from build123d import *

# Parameters (mm, degrees)
F1_DEPTH = 3.302
F2_DEPTH = 2.54
F3_R     = 5.715
F3_R_2   = 2.8702
F3_R_3   = 2.1123361497
F4_DEPTH = 3.303
F5_R     = 1.26999


# Not quite as in the source:
# - a fillet or chamfer is up to 0.001 mm smaller than in the source, because OpenCascade refuses the exact size


with BuildPart() as f1:
    # F0 (on Top) → F1 (new body)
    with BuildSketch(Plane.XY):
        with BuildLine():
            Line((86.5189202702, -3.8629329861), (10.3189202702, -3.8629329861))
            ThreePointArc((10.3189202702, -3.8629329861), (8.0738562399, -4.7928689558), (7.1439202702, -7.0379329861))
            Line((7.1439202702, -7.0379329861), (7.1439202702, -32.4379329861))
            ThreePointArc((7.1439202702, -32.4379329861), (8.0738562399, -34.6829970164), (10.3189202702, -35.6129329861))
            Line((10.3189202702, -35.6129329861), (86.5189202702, -35.6129329861))
            ThreePointArc((86.5189202702, -35.6129329861), (88.7639843005, -34.6829970164), (89.6939202702, -32.4379329861))
            Line((89.6939202702, -32.4379329861), (89.6939202702, -7.0379329861))
            ThreePointArc((89.6939202702, -7.0379329861), (88.7639843005, -4.7928689558), (86.5189202702, -3.8629329861))
        make_face()
        with BuildLine():
            Line((83.9789202702, -33.0729329861), (12.8589202702, -33.0729329861))
            ThreePointArc((12.8589202702, -33.0729329861), (10.6138562399, -32.1429970164), (9.6839202702, -29.8979329861))
            Line((9.6839202702, -29.8979329861), (9.6839202702, -9.5779329861))
            ThreePointArc((9.6839202702, -9.5779329861), (10.6138562399, -7.3328689558), (12.8589202702, -6.4029329861))
            Line((12.8589202702, -6.4029329861), (83.9789202702, -6.4029329861))
            ThreePointArc((83.9789202702, -6.4029329861), (86.2239843005, -7.3328689558), (87.1539202702, -9.5779329861))
            Line((87.1539202702, -9.5779329861), (87.1539202702, -29.8979329861))
            ThreePointArc((87.1539202702, -29.8979329861), (86.2239843005, -32.1429970164), (83.9789202702, -33.0729329861))
        make_face(mode=Mode.SUBTRACT)
        with BuildLine():
            ThreePointArc((9.6839202702, -29.8979329861), (10.6138562399, -32.1429970164), (12.8589202702, -33.0729329861))
            Line((12.8589202702, -33.0729329861), (83.9789202702, -33.0729329861))
            ThreePointArc((83.9789202702, -33.0729329861), (86.2239843005, -32.1429970164), (87.1539202702, -29.8979329861))
            Line((87.1539202702, -29.8979329861), (87.1539202702, -9.5779329861))
            ThreePointArc((87.1539202702, -9.5779329861), (86.2239843005, -7.3328689558), (83.9789202702, -6.4029329861))
            Line((83.9789202702, -6.4029329861), (12.8589202702, -6.4029329861))
            ThreePointArc((12.8589202702, -6.4029329861), (10.6138562399, -7.3328689558), (9.6839202702, -9.5779329861))
            Line((9.6839202702, -9.5779329861), (9.6839202702, -29.8979329861))
        make_face()
    extrude(amount=-F1_DEPTH)

    # F0 (on Top) → F2 (join)
    with BuildSketch(Plane.XY):
        with BuildLine():
            Line((86.5189202702, -3.8629329861), (10.3189202702, -3.8629329861))
            ThreePointArc((10.3189202702, -3.8629329861), (8.0738562399, -4.7928689558), (7.1439202702, -7.0379329861))
            Line((7.1439202702, -7.0379329861), (7.1439202702, -32.4379329861))
            ThreePointArc((7.1439202702, -32.4379329861), (8.0738562399, -34.6829970164), (10.3189202702, -35.6129329861))
            Line((10.3189202702, -35.6129329861), (86.5189202702, -35.6129329861))
            ThreePointArc((86.5189202702, -35.6129329861), (88.7639843005, -34.6829970164), (89.6939202702, -32.4379329861))
            Line((89.6939202702, -32.4379329861), (89.6939202702, -7.0379329861))
            ThreePointArc((89.6939202702, -7.0379329861), (88.7639843005, -4.7928689558), (86.5189202702, -3.8629329861))
        make_face()
        with BuildLine():
            Line((83.9789202702, -33.0729329861), (12.8589202702, -33.0729329861))
            ThreePointArc((12.8589202702, -33.0729329861), (10.6138562399, -32.1429970164), (9.6839202702, -29.8979329861))
            Line((9.6839202702, -29.8979329861), (9.6839202702, -9.5779329861))
            ThreePointArc((9.6839202702, -9.5779329861), (10.6138562399, -7.3328689558), (12.8589202702, -6.4029329861))
            Line((12.8589202702, -6.4029329861), (83.9789202702, -6.4029329861))
            ThreePointArc((83.9789202702, -6.4029329861), (86.2239843005, -7.3328689558), (87.1539202702, -9.5779329861))
            Line((87.1539202702, -9.5779329861), (87.1539202702, -29.8979329861))
            ThreePointArc((87.1539202702, -29.8979329861), (86.2239843005, -32.1429970164), (83.9789202702, -33.0729329861))
        make_face(mode=Mode.SUBTRACT)
    extrude(amount=F2_DEPTH)

    # F3 (on Top) → F4 (cut, through all)
    with BuildSketch(Plane.XY):
        with Locations((30.7151202702, -17.1979329861)):
            Circle(F3_R)
        with BuildLine():
            ThreePointArc((71.8377202702, -17.1979329861), (66.1227202702, -11.4829329861), (60.4077202702, -17.1979329861))
            ThreePointArc((60.4077202702, -17.1979329861), (66.1227202702, -22.9129329861), (71.8377202702, -17.1979329861))
        make_face()
        with Locations((43.1992202702, -13.949079439)):
            Circle(F3_R_2)
        with BuildLine():
            ThreePointArc((56.5088202702, -13.949079439), (53.6386202702, -11.078879439), (50.7684202702, -13.949079439))
            ThreePointArc((50.7684202702, -13.949079439), (53.6386202702, -16.819279439), (56.5088202702, -13.949079439))
        make_face()
        with Locations((48.4189202702, -22.2779329861)):
            Circle(F3_R_3)
    extrude(amount=-F4_DEPTH, mode=Mode.SUBTRACT)

    # F5 (radius 1.27 in the source; OpenCascade refuses exactly that, so slightly less here)
    f5_edges = [f1.edges().sort_by_distance(p)[0] for p in [
        (48.41892, -6.402933, 2.54),
        (10.613856, -7.332869, 2.54),
        (9.68392, -19.737933, 2.54),
        (10.613856, -32.142997, 2.54),
        (48.41892, -33.072933, 2.54),
        (87.15392, -19.737933, 2.54),
        (86.223984, -7.332869, 2.54),
        (86.223984, -32.142997, 2.54),
        (7.14392, -19.737933, 2.54),
        (8.073856, -4.792869, 2.54),
    ]]
    fillet(f5_edges, radius=F5_R)


solid = f1.part
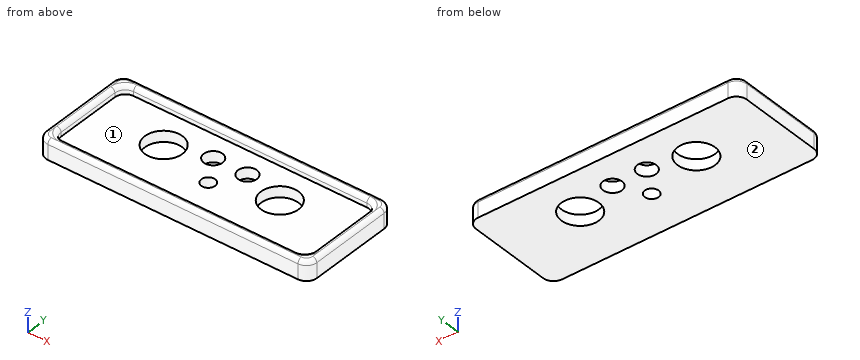
Geometry: final body of the model. Coordinates: model frame, mm. Face numbers are marked on the shaded views. Round coordinates to 2 decimals unless told otherwise and drop trailing zeros. Loops run counter-clockwise (first coordinate to the right, second up) from the corner with the lowest first, then second, coordinate; pieces in that order, holes last. Notation, with made-up numbers: (17, -30) -> (42, -30) arc R24 ccw to (42, 6) -> close; hole circle Ø1 at (-31, 38.25). An arc over 180 degrees is marked (long way). One line per question, with ' | ' between items. Start each with the question number.
1. Section B-B on z = -1.35. Output: boundary loops of the cut face in (x, y) (3 decimals), and give its area (3 significant figures).
2. Line query: line 1 along Y through (x, z) = (62.5, 0.5); line 2 along X through (y, z) = (-16, 0.1); line 3 along X through (y, z) = (-14, -2.95). Output: solid intervals per line, ascending. Write a range as [from, to].
3. Contact query for flat-ended pins moving along their axis: pin 1 (4 mm diameter, centred on x = 41.5, y = -17, fed in from +Z); pin 2 (10.5 mm diameter, centred on x = 30.72, y = -17.2, fed in from +Z). Output: stop coordinate, or through.
4. Mould query, pull axis Y, two halves, no side actions, for the marked faces 1 and 2. Classes: pulls with the +Y half, pulls with the -Y half, needs draft (parallel to the pull), parting line crosses it, or undercut.
5. Section C-C on y = -21.5. Count the separate pieces of the cut face and the enclosed holes in it, and give its area (3 significant figures).
Returned:
1) outline: (7.144, -32.438) arc R3.175 ccw to (10.319, -35.613) -> (86.519, -35.613) arc R3.175 ccw to (89.694, -32.438) -> (89.694, -7.038) arc R3.175 ccw to (86.519, -3.863) -> (10.319, -3.863) arc R3.175 ccw to (7.144, -7.038) -> close; hole circle Ø11.43 at (30.715, -17.198); hole circle Ø5.74 at (43.199, -13.949); hole circle Ø4.225 at (48.419, -22.278); hole circle Ø5.74 at (53.639, -13.949); hole circle Ø11.43 at (66.123, -17.198) | area: 2,340 mm2
2) line 1: y = [-35.61, -33.07], [-6.4, -3.86] | line 2: x = [7.14, 9.68], [87.15, 89.69] | line 3: x = [7.14, 25.98], [35.45, 40.33], [46.07, 50.77], [56.51, 61.39], [70.86, 89.69]
3) pin 1: stops at z = 0 | pin 2: passes through
4) face 1: undercut | face 2: needs draft
5) separate pieces: 4 | enclosed holes: 0 | area: 221 mm2
